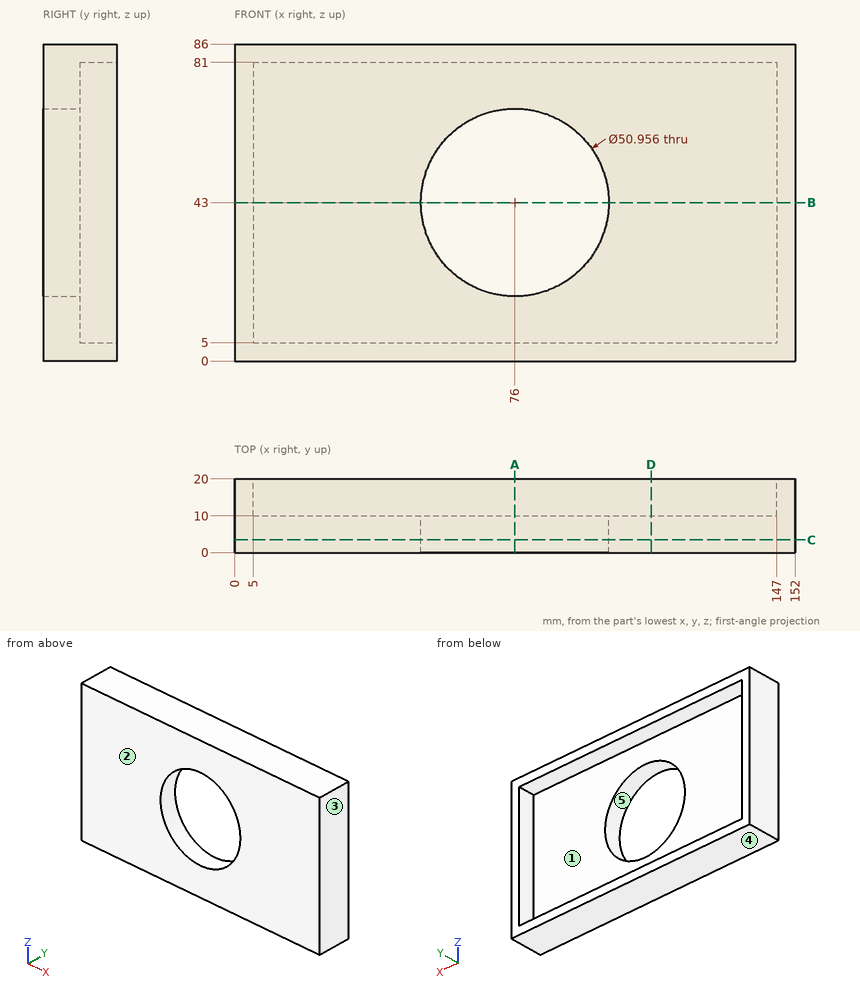
The drawing under review shows one solid part. Ordinate dimensions are in mm from its lowest x, y, z. A direction names the side the tool comes from. Coordinates: 2 decimals unless noted, no trailing zeros. Write each loop counter-clockwise with the first axis right and the second up, starting at its lowest first coordinate (ties: lowest second). Pieces come first, ordered by that corner, then holes. Notation, with made-up numbers: (27.5, 49) - (73.5, 49) arc R15 ccw to (73.5, 59) - close; hole circle Ø6 at (20, 37). An arc over 180 degrees is marked (long way). Answer as CSV lines item,"result".
(1) Mouldability with a two-part tool opening along Z and no side actions: class the marked faces 3, 4 and 5 as pulls with the +Z half, pulls with the -Z half, needs draft (parallel to the pull), parting line crosses it, or undercut.
Data:
face 3,"needs draft"
face 4,"pulls with the -Z half"
face 5,"undercut"
(2) We need section A-A (x = 76). Give the boundary of the cut face in (y, z).
Data:
outline,"(0, 0) - (20, 0) - (20, 5) - (10, 5) - (10, 17.52) - (0, 17.52) - close; (0, 68.48) - (10, 68.48) - (10, 81) - (20, 81) - (20, 86) - (0, 86) - close"
(3) We need section D-D (x = 113). Give the boundary of the cut face in (y, z).
Data:
outline,"(0, 0) - (20, 0) - (20, 5) - (10, 5) - (10, 81) - (20, 81) - (20, 86) - (0, 86) - close"
(4) Tool access review of the marked faces 1 and 2: name each direction out of +Z, -Z, +X, -X, +Y, -Y from which nothing blocks a thin tool from reaching the whole face with its end or side.
Data:
face 1,"+Y"
face 2,"+Z, -Z, +X, -X, -Y"
(5) We need section C-C (y = 3.5). Give the boundary of the cut face in (x, z) (1 decimal), plus the area to 3 significant figures.
Data:
outline,"(0, 0) - (152, 0) - (152, 86) - (0, 86) - close; hole circle Ø51 at (76, 43)"
area,"11,000 mm2"
(6) We need section B-B (z = 43). Give the boundary of the cut face in (x, y).
Data:
outline,"(0, 0) - (50.52, 0) - (50.52, 10) - (5, 10) - (5, 20) - (0, 20) - close; (101.48, 0) - (152, 0) - (152, 20) - (147, 20) - (147, 10) - (101.48, 10) - close"
(7) For line 1 along Z through (x, y) = (91, 12.75); line 2 along X through (y, z) = (12, 27.5); line 3 along Z through (x, y) = (76, 5), list the stretches that pass through material, from the lowest coordinate up. Write a range as [from, to].
Data:
line 1,"z = [0, 5], [81, 86]"
line 2,"x = [0, 5], [147, 152]"
line 3,"z = [0, 17.52], [68.48, 86]"
